from build123d import *

# Parameters (mm, degrees)
BOSS_EXTRUDE1_DEPTH = 2
FILLET1_R           = 0.1


with BuildPart() as part:
    # Sketch1 → Boss-Extrude1 (new body)
    with BuildSketch(Plane(origin=(0, 0, 0), x_dir=(1, 0, 0), z_dir=(0, 1, 0))):
        with BuildLine():
            Line((0.1, 40.499876543), (0.1, 37.499866666))
            ThreePointArc((0.1, 37.499866666), (26.551836095, 26.481125354), (37.5, 0))
            ThreePointArc((37.5, 0), (-26.481125354, -26.551836095), (-0.1, 37.499866666))
            Line((-0.1, 37.499866666), (-0.1, 40.499876543))
            ThreePointArc((-0.1, 40.499876543), (-28.602447448, -28.67315818), (40.5, 0))
            ThreePointArc((40.5, 0), (28.67315818, 28.602447448), (0.1, 40.499876543))
        make_face()
    extrude(amount=BOSS_EXTRUDE1_DEPTH)

    # Fillet1
    fillet1_edges = [part.edges().sort_by_distance(p)[0] for p in [
        (-0.1, 1, -37.499866666),
        (0.1, 1, -37.499866666),
        (0.1, 1, -40.499876543),
        (-0.1, 1, -40.499876543),
    ]]
    fillet(fillet1_edges, radius=FILLET1_R)


solid = part.part
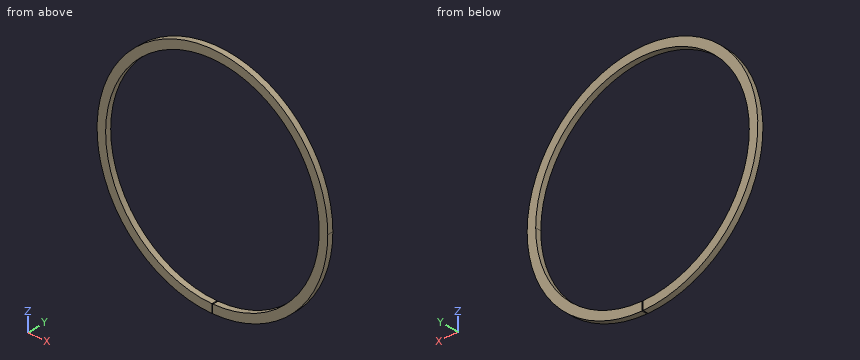
Verification items for the finished model (mm, model axes). Give positions to 0.01 mm unless a question says otherwise; leave off trailing zeros. Write each loop counter-clockwise with the first axis right and the second up, starting at its lowest first coordinate (ties: lowest second). Pieces come first, ordered by that corner, then holes. Notation, with made-up numbers: M 86,69.25 L 135,69.25 A19 ccw 135,98.25 Z; hole C 47,-30 d10. An arc over 180 degrees is marked long. Put each result on its own line as item: value. Start each with the question number.
1. Section check A-A (x = 30). Record the cut outline in (y, z).
2. Scan lines: line 1 along Z through (x, y) = (24, 0.1); line 2 along X through (y, z) = (1.65, -30); line 3 along Z through (x, y) = (0, 1.05). Record each from-to range of solid material in increasing order. Write a range as [from, to].
3. Section check B-B (z = -21.5). Record the cut outline in (x, y).
4. Section check C-C (y = 1). Record the cut outline in (x, z).
Answer list:
1. outline: M 0,-27.21 L 2,-27.21 L 2,-22.5 L 0,-22.5 Z; M 0,22.5 L 2,22.5 L 2,27.21 L 0,27.21 Z
2. line 1: [-32.62, -28.81], [28.81, 32.62]
2. line 2: [-27.21, -22.5], [22.5, 27.21]
2. line 3: [37.5, 40.5]
3. outline: M -34.32,0 L -30.72,0 L -30.72,2 L -34.32,2 Z; M 30.72,0 L 34.32,0 L 34.32,2 L 30.72,2 Z
4. outline: M -0.2,-40.5 A0.1 ccw -0.1,-40.4 L -0.1,-37.6 A0.1 ccw -0.2,-37.5 A37.5 cw long 0.2,-37.5 A0.1 ccw 0.1,-37.6 L 0.1,-40.4 A0.1 ccw 0.2,-40.5 A40.5 ccw long Z
